Geometry check sheet. Reference: the model listing, model coordinates, mm. Face numbers are marked on the shaded views. Give positions to 0.01 mm unless a question says otherwise; leave off trailing zeros. Order: outer loops, then holes, each group sorted by start corner. A loop starts at its lowest first (then second) coordinate and runs counter-clockwise, first axis right, second up. Notation, with made-up numbers: M 55.5,63.5 L 93.5,63.5 A7 ccw 93.5,67.5 Z; hole C 21.5,-6.75 d5. An arc over 180 degrees is marked long. Put each result on its own line as item: value. Start each with the question number.
Q1. Section check A-A on y = 5. Record the cut outline in (x, z).
Q2. Mould release check, pull along Z, two halves, no side actions. Record for the marked faces 1, 2 and 3: +Z half, -Z half, draft (parallel to the pull), parting line (faces both ways), or undercut.
Q3. Section check C-C on z = -0.5. Record the cut outline in (x, y), then the cut area to 3 significant figures.
Q4. Section check B-B on x = 15. Record the cut outline in (y, z), then the cut area to 3 significant figures.
Q5. Material ranges on L1, parallel to Z at x = 19.5, y = 6.25; L2, parallel to Y at x = -53, z = 6.5; L3, parallel to X at y = 9.75, z = -11.5, recorded low to high.
Q6. Go/stop test with flat-tipped pins: pin 1 (4 mm diameter, centred on y = 10, z = 6, fed in from +X); pin 2 (5 mm diameter, centred on x = 7.5, y = 4, fed in from -Z); pin 3 (10.5 mm diameter, centred on x = -9.5, z = -1, fed in from -Y). Record where each tip stops, or that it passes through.
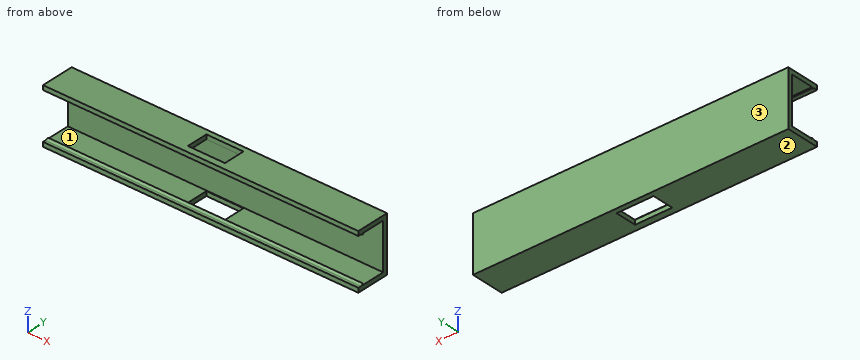
```python
from build123d import *

# Parameters (mm, degrees)
CROQUIS1_W              = 142
CROQUIS1_H              = 20.7
CROQUIS1_H_2            = 2.15
SALIENTE_EXTRUIR1_DEPTH = 15
CROQUIS2_W              = 21
CROQUIS2_H              = 13
CORTAR_EXTRUIR1_DEPTH   = 230
SALIENTE_EXTRUIR4_DEPTH = 142
CROQUIS12_W             = 16.7
CROQUIS12_H             = 9.7
CORTAR_EXTRUIR2_DEPTH   = 50


with BuildPart() as part:
    # Croquis1 → Saliente-Extruir1 (new body)
    with BuildSketch(Plane(origin=(0, 0, 0), x_dir=(1, 0, 0), z_dir=(0, 1, 0))):
        Rectangle(CROQUIS1_W, CROQUIS1_H)
        with Locations((0, 11.425)):
            Rectangle(CROQUIS1_W, CROQUIS1_H_2)
        with Locations((0, -11.425)):
            Rectangle(CROQUIS1_W, CROQUIS1_H_2)
    extrude(amount=SALIENTE_EXTRUIR1_DEPTH)

    # Croquis2 → Cortar-Extruir1 (cut)
    with BuildSketch(Plane.ZY.offset(71)):
        with Locations((0, 6.5)):
            Rectangle(CROQUIS2_W, CROQUIS2_H)
    extrude(amount=-CORTAR_EXTRUIR1_DEPTH, mode=Mode.SUBTRACT)

    # Croquis11 → Saliente-Extruir4 (add)
    with BuildSketch(Plane.ZY.offset(71)):
        Polygon((-10.5, 1.35), (-10.5, 2.55), (-10, 2.55), align=None)
        Polygon((10, 2.55), (10.5, 1.35), (10.5, 2.55), align=None)
    extrude(amount=-SALIENTE_EXTRUIR4_DEPTH)

    # Croquis12 → Cortar-Extruir2 (cut)
    with BuildSketch(Plane.XY.offset(12.5)):
        with Locations((0, 7.85)):
            Rectangle(CROQUIS12_W, CROQUIS12_H)
    extrude(amount=-CORTAR_EXTRUIR2_DEPTH, mode=Mode.SUBTRACT)


solid = part.part
```
Results found:
1. outline: M -71,-12.5 L -8.35,-12.5 L -8.35,-10.5 L -71,-10.5 Z; M -71,10.5 L -8.35,10.5 L -8.35,12.5 L -71,12.5 Z; M 8.35,-12.5 L 71,-12.5 L 71,-10.5 L 8.35,-10.5 Z; M 8.35,10.5 L 71,10.5 L 71,12.5 L 8.35,12.5 Z
2. face 1: undercut
2. face 2: -Z half
2. face 3: draft
3. outline: M -71,13 L 71,13 L 71,15 L -71,15 Z
3. area: 284 mm^2
4. outline: M 0,-12.5 L 15,-12.5 L 15,12.5 L 0,12.5 L 0,10.5 L 1.35,10.5 L 2.55,10 L 2.55,10.5 L 13,10.5 L 13,-10.5 L 2.55,-10.5 L 2.55,-10 L 1.35,-10.5 L 0,-10.5 Z
4. area: 103 mm^2
5. L1: z = -12.5 to -10.5, 10.5 to 12.5
5. L2: y = 13 to 15
5. L3: x = -71 to -8.35, 8.35 to 71
6. pin 1: passes through
6. pin 2: stops at z = -12.5
6. pin 3: stops at y = 13
